Source: CAD feature listing. Evaluate the final solid. Frame: model axes, mm. Face numbers are marked on the shaded views. A direction names the side the tool comes from. Give positions to 0.01 mm unless a question says otherwise; leave off trailing zeros. Write each loop counter-clockwise with the first axis right and the second up, starting at its lowest first coordinate (ties: lowest second). Pieces come first, ordered by that corner, then holes. Notation, with made-up numbers: (70.5, 0) - (107.5, 0) arc R20 cw to (107.5, 30) - close; hole circle Ø9 at (-19.5, -19.5). An arc over 180 degrees is marked (long way). One line per question, with ' | ' between items. Start each with the question number.
(1) Pin query (flat end, axial travel): pin 1 (5 mm diameter, centred on x = 8.5, z = -5, fed in from -Y); pin 2 (1 mm diameter, centred on x = -9, z = 1, fed in from -Y); pin 3 (1.2 mm diameter, centred on x = -3.5, y = -4.5, fed in from +Z). Return the tip coordinate at first contact, or that it passes through.
(2) Section B-B, the plane y = 0. Return loops of the section in (x, z), plus the area to 3 significant figures.
(3) Section A-A, the plane z = 2.25. Return loops of the section in (x, y).
(4) Draft query along Y for the marked faces 1, 2 and 3. Return one class per face: +Y half, -Y half, draft (parallel to the pull), parting line (faces both ways), or undercut.
(5) Ray query, line 1 (Y direction, x = 9.9, z = 0.4); line 2 (Z direction, x = -3.25, y = 3.75); line 3 (X direction, y = 1.25, z = 2.75). Return the intervals inside material, ascending. Write a range as [from, to].
(6) Section C-C, the plane z = -5.25. Return loops of the section in (x, y).
(7) Section D-D, the plane x = 1.37. Return loops of the section in (y, z).
(8) Access query for the marked faces 4, 5 and 6. Directions: +Z, -Z, +X, -X, +Y, -Y. A direction counts if a zero-diameter tool reaches every point of the face in a straight line with its end or side. Return the directions, or none.
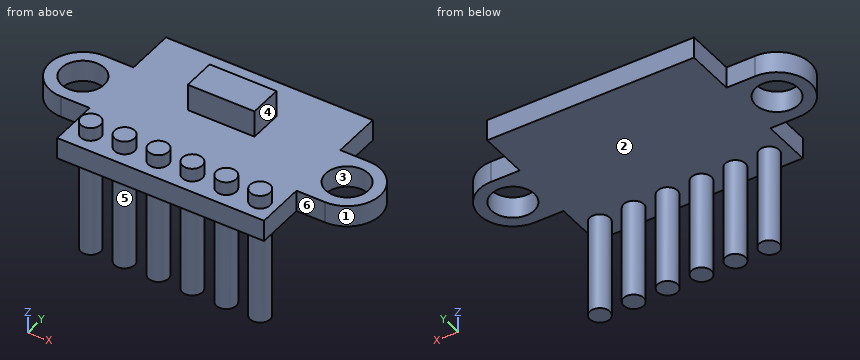
```python
from build123d import *

# Parameters (mm, degrees)
SKETCH1_R       = 1.6
MAIN_DEPTH      = 1.6
SKETCH2_W       = 5
SKETCH2_H       = 2.5
SENSOR_DEPTH    = 2
SKETCH3_R       = 0.75
CABLES_DEPTH    = 10
LPATTERN1_COUNT = 6
LPATTERN1_PITCH = 2.54


with BuildPart() as part:
    # Sketch1 → Main (new body)
    with BuildSketch(Plane.XY):
        with BuildLine():
            Line((-7.75, 6.2), (7.75, 6.2))
            Line((7.75, 6.2), (7.75, 2.5))
            Line((7.75, 2.5), (9.9, 2.5))
            ThreePointArc((9.9, 2.5), (12.4, 0), (9.9, -2.5))
            Line((9.9, -2.5), (7.75, -2.5))
            Line((7.75, -2.5), (7.75, -6.2))
            Line((7.75, -6.2), (-7.75, -6.2))
            Line((-7.75, -6.2), (-7.75, -2.5))
            Line((-7.75, -2.5), (-9.9, -2.5))
            ThreePointArc((-9.9, -2.5), (-12.4, 0), (-9.9, 2.5))
            Line((-9.9, 2.5), (-7.75, 2.5))
            Line((-7.75, 2.5), (-7.75, 6.2))
        make_face()
        with Locations((-9.9, 0)):
            Circle(SKETCH1_R, mode=Mode.SUBTRACT)
        with Locations((9.9, 0)):
            Circle(SKETCH1_R, mode=Mode.SUBTRACT)
    extrude(amount=MAIN_DEPTH)

    # Sketch2 → Sensor (add)
    with BuildSketch(Plane.XY.offset(1.6)):
        with Locations((0, 1.95)):
            Rectangle(SKETCH2_W, SKETCH2_H)
    extrude(amount=SENSOR_DEPTH)

    # Sketch3 → Cables (add)
    with BuildSketch(Plane.XY.offset(2.6)):
        with Locations((-6.25, -4.66)):
            Circle(SKETCH3_R)
    cables = extrude(amount=-CABLES_DEPTH)

    # LPattern1: Cables ×6
    with Locations(*[(i * LPATTERN1_PITCH, 0, 0) for i in range(1, LPATTERN1_COUNT)]):
        add(cables)


solid = part.part
```
Check sheet entries:
1) pin 1: y = -5.41 | pin 2: y = -2.5 | pin 3: z = 2.6
2) outline: (-12.4, 0) - (-11.5, 0) - (-11.5, 1.6) - (-12.4, 1.6) - close; (-8.3, 0) - (8.3, 0) - (8.3, 1.6) - (-8.3, 1.6) - close; (11.5, 0) - (12.4, 0) - (12.4, 1.6) - (11.5, 1.6) - close | area: 29.4 mm²
3) outline: circle Ø1.5 at (-6.25, -4.66); circle Ø1.5 at (-3.71, -4.66); (-2.5, 0.7) - (2.5, 0.7) - (2.5, 3.2) - (-2.5, 3.2) - close; circle Ø1.5 at (-1.17, -4.66); circle Ø1.5 at (1.37, -4.66); circle Ø1.5 at (3.91, -4.66); circle Ø1.5 at (6.45, -4.66)
4) face 1: parting line | face 2: draft | face 3: undercut
5) line 1: [-2.5, -1.6], [1.6, 2.5] | line 2: [0, 1.6] | line 3: [-2.5, 2.5]
6) outline: circle Ø1.5 at (-6.25, -4.66); circle Ø1.5 at (-3.71, -4.66); circle Ø1.5 at (-1.17, -4.66); circle Ø1.5 at (1.37, -4.66); circle Ø1.5 at (3.91, -4.66); circle Ø1.5 at (6.45, -4.66)
7) outline: (-6.2, 0) - (-5.41, 0) - (-5.41, -7.4) - (-3.91, -7.4) - (-3.91, 0) - (6.2, 0) - (6.2, 1.6) - (3.2, 1.6) - (3.2, 3.6) - (0.7, 3.6) - (0.7, 1.6) - (-3.91, 1.6) - (-3.91, 2.6) - (-5.41, 2.6) - (-5.41, 1.6) - (-6.2, 1.6) - close
8) face 4: +Z, +X, +Y, -Y | face 5: -Z | face 6: +Z, -Z, +X, -Y
